For this review, take the finished solid that the model builds, in its own axes (mm). A direction names the side the tool comes from. Round coordinates to 2 decimals unless told otherwise and drop trailing zeros. Write each loop counter-clockwise with the first axis right and the second up, starting at its lowest first coordinate (ties: lowest second). Pieces come first, ordered by that corner, then holes. Notation, with made-up numbers: (64.5, -9.5) -> (94.5, -9.5) arc R16 cw to (94.5, 3.5) -> close; hole circle Ø4 at (-5, 58). An arc over 180 degrees is marked (long way). Answer in a Markdown table with one row per item.
from build123d import *

# Parameters (mm, degrees)
SKETCH_1_W          = 13.2
SKETCH_1_H          = 20
EXTRUDE_1_DEPTH     = 2
SKETCH_1_3_R        = 0.75
CUT_EXTRUDE_2_DEPTH = 13.147427711
CUT_EXTRUDE_START   = -2
SKETCH_2_W          = 10.3
SKETCH_2_H          = 3.5
CUT_EXTRUDE_1_DEPTH = 1
SKETCH_2_3_R        = 0.7
CUT_EXTRUDE_4_DEPTH = 13.147427711


with BuildPart() as part:
    # 草图1 → 凸台-拉伸1 (new body)
    with BuildSketch(Plane(origin=(0, 0, 0), x_dir=(1, 0, 0), z_dir=(0, 1, 0))):
        Rectangle(SKETCH_1_W, SKETCH_1_H)
    extrude(amount=EXTRUDE_1_DEPTH)

    # 草图1<3> → 切除-拉伸2 (cut, through all)
    with BuildSketch(Plane(origin=(0, 0, 0), x_dir=(1, 0, 0), z_dir=(0, 1, 0))):
        with Locations(Location((-5.2, -8.6, 0), (0, 0, 270))):
            Circle(SKETCH_1_3_R)
        with Locations(Location((5.2, 8.6, 0), (0, 0, 270))):
            Circle(SKETCH_1_3_R)
    extrude(amount=CUT_EXTRUDE_2_DEPTH, mode=Mode.SUBTRACT)

    # 草图2 → 切除-拉伸1 (cut)
    with BuildSketch(Plane(origin=(0, 2, 0), x_dir=(1, 0, 0), z_dir=(0, 1, 0)).offset(CUT_EXTRUDE_START)):
        with Locations((-1.45, 8.25)):
            Rectangle(SKETCH_2_W, SKETCH_2_H)
        with Locations((1.45, -8.25)):
            Rectangle(SKETCH_2_W, SKETCH_2_H)
    extrude(amount=CUT_EXTRUDE_1_DEPTH, mode=Mode.SUBTRACT)

    # 草图2<3> → 切除-拉伸4 (cut, through all)
    with BuildSketch(Plane(origin=(0, 2, 0), x_dir=(1, 0, 0), z_dir=(0, 1, 0))):
        with Locations(Location((-2.6, -8.75, 0), (0, 0, 270))):
            Circle(SKETCH_2_3_R)
        with Locations(Location((2.4, -8.75, 0), (0, 0, 270))):
            Circle(SKETCH_2_3_R)
        with Locations(Location((-2.4, 8.5, 0), (0, 0, 270))):
            Circle(SKETCH_2_3_R)
        with Locations(Location((2.6, 8.5, 0), (0, 0, 270))):
            Circle(SKETCH_2_3_R)
    extrude(amount=-CUT_EXTRUDE_4_DEPTH, mode=Mode.SUBTRACT)


solid = part.part
1) Consider section A-A on y = 1.8. State the section outline as (x, z) points.
Solved:
| item | result |
|---|---|
| outline | (-6.6, -10) -> (6.6, -10) -> (6.6, 10) -> (-6.6, 10) -> close; hole circle Ø1.5 at (-5.2, 8.6); hole circle Ø1.4 at (-2.6, 8.75); hole circle Ø1.4 at (-2.4, -8.5); hole circle Ø1.4 at (2.4, 8.75); hole circle Ø1.4 at (2.6, -8.5); hole circle Ø1.5 at (5.2, -8.6) |
2) Mouldability with a two-part tool opening along X and no side actions: class faces 1 (the flat face through (-6.6, 1, 0)), 2 (the cylindrical face through (-2.4, 1.5, -9.2)), 3 (the flat face through (1, 1, 8)) as pulls with the +X half, pulls with the -X half, needs draft (parallel to the pull), parting line crosses it, or undercut.
Solved:
| item | result |
|---|---|
| face 1 | pulls with the -X half |
| face 2 | undercut |
| face 3 | needs draft |
3) Consider section B-B on x = 5.2. State the section outline as (y, z) points, then the cut area to 3 significant figures.
Solved:
| item | result |
|---|---|
| outline | (0, -10) -> (2, -10) -> (2, -9.35) -> (0, -9.35) -> close; (0, -7.85) -> (2, -7.85) -> (2, 10) -> (1, 10) -> (1, 6.5) -> (0, 6.5) -> close |
| area | 33.5 mm² |
4) Consider section D-D on y = 0.25. State the section outline as (x, z) points.
Solved:
| item | result |
|---|---|
| outline | (-6.6, -6.5) -> (3.7, -6.5) -> (3.7, -10) -> (6.6, -10) -> (6.6, 6.5) -> (-3.7, 6.5) -> (-3.7, 10) -> (-6.6, 10) -> close; hole circle Ø1.5 at (-5.2, 8.6); hole circle Ø1.5 at (5.2, -8.6) |
5) Clearance check with flat-ended pins moving along their axes: pin 1 Ø0.8 at (x, y) = (-0.5, 0.5) entering from +Z; pin 2 Ø0.8 at (y, z) = (0.5, -7.5) entering from -X. State where each tip first meets the part, or that it passes through.
Solved:
| item | result |
|---|---|
| pin 1 | z = 6.5 |
| pin 2 | x = 3.7 |
6) Consider section C-C on z = -8.6. State the section outline as (x, y) points, then the cut area to 3 significant figures.
Solved:
| item | result |
|---|---|
| outline | (-6.6, 1) -> (-3.09, 1) -> (-3.09, 2) -> (-6.6, 2) -> close; (-1.71, 1) -> (1.91, 1) -> (1.91, 2) -> (-1.71, 2) -> close; (3.29, 1) -> (3.7, 1) -> (3.7, 0) -> (4.45, 0) -> (4.45, 2) -> (3.29, 2) -> close; (5.95, 0) -> (6.6, 0) -> (6.6, 2) -> (5.95, 2) -> close |
| area | 10.3 mm² |
7) For line 1 (X direction, y = 1.2, z = 8.75); line 2 (Z direction, x = -2, y = 1.55); line 3 (Z direction, x = -2.75, y = 0.25), list the stretches that pass through material, from the lowest coordinate up. Write a range as [from, to].
Solved:
| item | result |
|---|---|
| line 1 | [-6.6, -5.93], [-4.47, -3.3], [-1.9, 1.7], [3.1, 6.6] |
| line 2 | [-10, -9.07], [-7.93, 8.39], [9.11, 10] |
| line 3 | [-6.5, 6.5] |
8) For faces 4 (the flat face through (-1.5, 0.5, -6.5)), 5 (the flat face through (-3.7, 0.5, 8.3)), 6 (the cylindrical face through (2.174, 1.507, -9.055)), list the 3-axis set-ups (+Z, -Z, +X, -X, +Y, -Y) from which the entire face can be reached by the end or side of a thin tool; tool diameter is ignored.
Solved:
| item | result |
|---|---|
| face 4 | -Z, -X, -Y |
| face 5 | +Z, +X, -Y |
| face 6 | +Y, -Y |
